Can you work these out from the model? Positions are in its coordinate system, mm. A direction names the side the tool comes from. Give positions to 0.01 mm unless a question says otherwise; leave off trailing zeros. Loops run counter-clockwise (first coordinate to the right, second up) from the corner with the lowest first, then second, coordinate; pieces in that order, holes last. Notation, with made-up numbers: M 81.5,7.5 L 88.5,7.5 A17 cw 88.5,33.5 Z; hole C 4,-8.5 d10. An arc over 180 degrees is marked long. Answer as a JSON object with one key per item and string values.
```python
from build123d import *

# Parameters (mm, degrees)
F1_DEPTH = 15
F2_DEPTH = 2


with BuildPart() as f1:
    # F0 (on Top) → F1 (new body)
    with BuildSketch(Plane.XY):
        with BuildLine():
            ThreePointArc((-20.774407, 2.498756), (-23.346099, 0.18924), (-21.152519, -2.482026))
            ThreePointArc((-21.152519, -2.482026), (-19.194675, -1.870577), (-18.353272, 0))
            ThreePointArc((-18.353272, 0), (-19.057839, 1.739661), (-20.774407, 2.498756))
        make_face()
    extrude(amount=F1_DEPTH)

    # F0 (on Top) → F2 (join)
    with BuildSketch(Plane.XY):
        with BuildLine():
            Line((-21.152519, -2.482026), (-0.793802, -4.936586))
            Line((-0.793802, -4.936586), (-0.402254, -4.983793))
            ThreePointArc((-0.402254, -4.983793), (4.999974, -0.016188), (-0.369976, 4.986293))
            Line((-0.369976, 4.986293), (-0.83883, 4.929134))
            Line((-0.83883, 4.929134), (-20.774407, 2.498756))
            ThreePointArc((-20.774407, 2.498756), (-19.057839, 1.739661), (-18.353272, 0))
            ThreePointArc((-18.353272, 0), (-19.194675, -1.870577), (-21.152519, -2.482026))
        make_face()
        with BuildLine():
            ThreePointArc((0.65, 2.672078), (2.162175, 1.699265), (2.75, 0))
            ThreePointArc((2.75, 0), (2.162175, -1.699265), (0.65, -2.672078))
            ThreePointArc((0.65, -2.672078), (0, -2.75), (-0.65, -2.672078))
            ThreePointArc((-0.65, -2.672078), (-2.75, 0), (-0.65, 2.672078))
            ThreePointArc((-0.65, 2.672078), (0, 2.75), (0.65, 2.672078))
        make_face(mode=Mode.SUBTRACT)
        with BuildLine():
            Line((0.65, -2.672078), (0.65, 2.672078))
            ThreePointArc((0.65, 2.672078), (0, 2.75), (-0.65, 2.672078))
            Line((-0.65, 2.672078), (-0.65, -2.672078))
            ThreePointArc((-0.65, -2.672078), (0, -2.75), (0.65, -2.672078))
        make_face()
    extrude(amount=F2_DEPTH)


solid = f1.part
```
1) For faces 1 (the flat face through (-21, 0, 15)), 2 (the flat face through (0.65, 0, 1)), which set-ups out of +Z, -Z, +X, -X, +Y, -Y let a thin tool reach every point of the face, with its end or its side?
Answer list:
{"face 1": "+Z, +X, -X, +Y, -Y", "face 2": "+Z, -Z"}
2) Will these pins go through, and if not, where does the flat tip stop? pin 1 Ø8 at (x, z) = (-17, 4) entering from +Y; pin 2 Ø1 at (x, z) = (-17, 8.5) entering from -Y; pin 3 Ø1 at (y, z) = (1.5, 1) entering from -X; pin 4 Ø1.5 at (x, y) = (-9, 1.5) entering from +Z.
Answer list:
{"pin 1": "y = 3.38", "pin 2": "through", "pin 3": "x = -23.14", "pin 4": "z = 2"}
3) If we mould it in two halves opening along Y, with no side actions, what happens to faces 3 (the flat face through (-0.65, 0, 1)), 4 (the flat face through (-5, 0, 2)), 5 (the cylindrical face through (5, 0, 1))? For each: +Y half, -Y half, draft (parallel to the pull), parting line (faces both ways), or undercut.
Answer list:
{"face 3": "undercut", "face 4": "draft", "face 5": "parting line"}
4) Suppose I cut it at B-B, the plane x = 0. Write out the boundary of the cut face in (y, z), and give its area (3 significant figures).
Answer list:
{"outline": "M -5,0 L 5,0 L 5,2 L -5,2 Z", "area": "20.0 mm^2"}
5) Please list where these lines run through material, in increasing order: line 1 along X through (y, z) = (-1.75, 1.75); line 2 along Z through (x, y) = (-17.25, 2); line 3 along X through (y, z) = (-2, 1.25). Write a range as from..to.
Answer list:
{"line 1": "-22.64..-2.12, -0.65..0.65, 2.12..4.68", "line 2": "0..2", "line 3": "-22.35..-1.89, -0.65..0.65, 1.89..4.58"}
6) Suppose I cut it at D-D, the plane y = 4.5. Write out the boundary of the cut face in (x, z).
Answer list:
{"outline": "M -4.36,0 L 2.18,0 L 2.18,2 L -4.36,2 Z"}
7) Suppose I cut it at C-C, the plane z = 12. Write out the boundary of the cut face in (x, y).
Answer list:
{"outline": "M -20.77,2.5 A2.5 ccw long -18.35,0 A2.5 ccw Z"}
8) Suppose I cut it at A-A, the plane y = -1.5. Write out the boundary of the cut face in (x, z).
Answer list:
{"outline": "M -22.85,0 L -2.3,0 L -2.3,2 L -18.85,2 L -18.85,15 L -22.85,15 Z; M -0.65,0 L 0.65,0 L 0.65,2 L -0.65,2 Z; M 2.3,0 L 4.77,0 L 4.77,2 L 2.3,2 Z"}
